Design review of the part built by this model. Coordinates are the model's own, in mm. A direction names the side the tool comes from. Coordinates: 2 decimals unless noted, no trailing zeros. Order: outer loops, then holes, each group sorted by start corner. A loop starts at its lowest first (then second) coordinate and runs counter-clockwise, first axis right, second up. Notation, with made-up numbers: M -38.75,1 L 8.25,1 A8 ccw 8.25,10 Z; hole C -32.5,-25.5 d2. An arc over 180 degrees is marked long. Use CSV: the item, a comma, the result in double quotes.
```python
from build123d import *

# Parameters (mm, degrees)
F0_R     = 23.9192744627
F1_DEPTH = 151.98784
F2_R     = 19.4620024737
F3_DEPTH = 219.48349
F4_T     = -2.54


with BuildPart() as f1:
    # F0 (on Front) → F1 (new body)
    with BuildSketch(Plane.XZ):
        Circle(F0_R)
    extrude(amount=F1_DEPTH)

    # F2 (on face) → F3 (join)
    with BuildSketch(Plane.XZ.offset(151.98784)):
        Circle(F2_R)
    extrude(amount=-F3_DEPTH)

    # F4
    f4_openings = [f1.faces().sort_by_distance(p)[0] for p in [
        (0, -151.98784, 0),
    ]]
    offset(amount=F4_T, openings=f4_openings, kind=Kind.INTERSECTION)


solid = f1.part
```
(1) The part is to be moulded in two halves that separate along Z. For faces 1 (the face through (0, 64.956, 0)), 2 (the face through (0, 67.496, 0)), 3 (the face through (-5.19, -74.93, -23.35)), say which applies: pulls with the +Z half, pulls with the -Z half, needs draft (parallel to the pull), parting line crosses it, or undercut.
The answers:
face 1,"undercut"
face 2,"needs draft"
face 3,"parting line crosses it"
(2) Add section A-A on y = 16.5. State the section outline as (x, z) points.
The answers:
outline,"C 0,0 d38.92; hole C 0,0 d33.84"
(3) Clearance check with flat-ended pins moving along their axes: P1, Ø4, axis at x = 10, y = -101.5, coming from the +Z side; P2, Ø21.5, axis at x = 0.5, z = 4.5, coming from the -Y side; P3, Ø4, axis at x = -8.5, z = -15.5, coming from the -Y side. State where each tip first meets the part, or that it passes through.
The answers:
P1,"stops at z = 22.54"
P2,"stops at y = 64.96"
P3,"stops at y = -2.54"
(4) Add section C-C on x = 0. State the section outline as (y, z) points.
The answers:
outline,"M -151.99,-23.92 L 0,-23.92 L 0,-19.46 L 67.5,-19.46 L 67.5,19.46 L 0,19.46 L 0,23.92 L -151.99,23.92 L -151.99,21.38 L -2.54,21.38 L -2.54,16.92 L 64.96,16.92 L 64.96,-16.92 L -2.54,-16.92 L -2.54,-21.38 L -151.99,-21.38 Z"
(5) Wall thickness on probe 1 along Z at (x, y) = (0, -72); probe 2 along Y at (x, z) = (-14.5, 14); probe 3 along Y at (x, z) = (13, 17): over which ranges is each line inside the solid? List them lowest first.
The answers:
probe 1,"z = -23.92 to -21.38, 21.38 to 23.92"
probe 2,"y = -2.54 to 0"
probe 3,"y = -151.99 to 0"
(6) Add section B-B on z = 0. State the section outline as (x, y) points, and give its area (3 significant figures).
The answers:
outline,"M -23.92,-151.99 L -21.38,-151.99 L -21.38,-2.54 L -16.92,-2.54 L -16.92,64.96 L 16.92,64.96 L 16.92,-2.54 L 21.38,-2.54 L 21.38,-151.99 L 23.92,-151.99 L 23.92,0 L 19.46,0 L 19.46,67.5 L -19.46,67.5 L -19.46,0 L -23.92,0 Z"
area,"1,220 mm2"
(7) For faces 4 (the face through (-4.22, 33.28, -19)), 5 (the face through (-18, -151.988, -12)), 6 (the face through (16, -2.54, 6)), list the 3-axis set-ups (+Z, -Z, +X, -X, +Y, -Y) from which the entire face can be reached by the end or side of a thin tool; tool diameter is ignored.
The answers:
face 4,"+Y"
face 5,"+Z, -Z, +X, -X, -Y"
face 6,"-Y"
(8) Add section D-D on y = -103.5. State the section outline as (x, z) points.
The answers:
outline,"C 0,0 d47.84; hole C 0,0 d42.76"
